```python
from build123d import *

# Parameters (mm, degrees)
F0_R     = 1.494135
F1_DEPTH = 2.54


with BuildPart() as f1:
    # F0 (on Top) → F1 (new body)
    with BuildSketch(Plane.XY):
        with BuildLine():
            Line((13.48222, 2.024483), (3.201543, 2.496718))
            Line((3.201543, 2.496718), (0.474253, 11.350792))
            ThreePointArc((0.474253, 11.350792), (0.005987, 16.463631), (-0.486017, 11.353022))
            Line((-0.486017, 11.353022), (-3.337723, 2.332209))
            Line((-3.337723, 2.332209), (-13.398782, 1.982259))
            Line((-13.398782, 1.982259), (-5.530131, -4.593079))
            Line((-5.530131, -4.593079), (-8.383425, -15.383421))
            Line((-8.383425, -15.383421), (-8.195174, -15.200495))
            Line((-8.195174, -15.200495), (0, -9.12891))
            Line((0, -9.12891), (8.333031, -15.200495))
            Line((8.333031, -15.200495), (5.491082, -4.593079))
            Line((5.491082, -4.593079), (5.580035, -4.494939))
            Line((5.580035, -4.494939), (13.48222, 2.024483))
        make_face()
        Polygon((-0.515748, -8.972427), (-7.396878, -14.017268), (-0.785596, -2.886029), (-0.214107, -8.758916), align=None, mode=Mode.SUBTRACT)
        Polygon((-12.247529, 1.427319), (-1.096065, -2.263094), (-5.187609, -4.228639), align=None, mode=Mode.SUBTRACT)
        Polygon((4.948679, -4.494939), (7.647161, -14.017268), (0, -2.683643), align=None, mode=Mode.SUBTRACT)
        Polygon((11.950911, 1.767228), (0, -1.88404), (3.035744, 1.982259), align=None, mode=Mode.SUBTRACT)
        Polygon((-2.941626, 2.241765), (-0.236567, 11.293307), (-0.65273, -1.555721), align=None, mode=Mode.SUBTRACT)
        with Locations((0, 13.88522)):
            Circle(F0_R, mode=Mode.SUBTRACT)
    extrude(amount=F1_DEPTH)


solid = f1.part
```
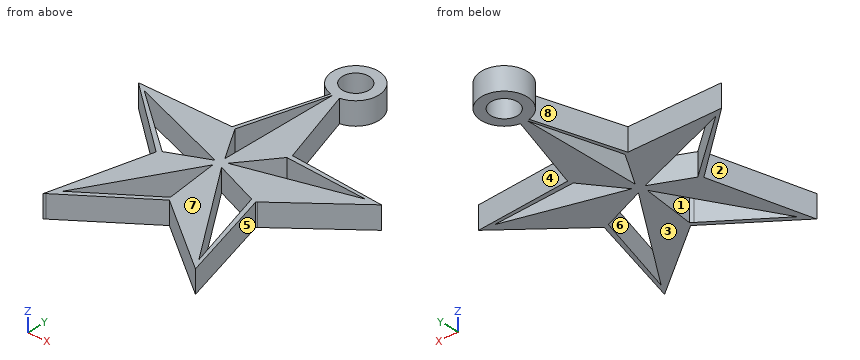
Can you work these out from the model? Positions are in its coordinate system, mm. Face numbers are marked on the shaded views. A direction names the side the tool comes from. Coordinates: 2 decimals unless noted, no trailing zeros. Loops run counter-clockwise (first coordinate to the right, second up) from the corner with the lowest first, then second, coordinate; pieces in that order, holes last. Notation, with made-up numbers: (-25.75, -34.75) -> (24.25, -34.75) arc R17 ccw to (24.25, -18.75) -> close; hole circle Ø4 at (-3.75, 56). An arc over 180 degrees is marked (long way). Answer as a JSON object with one key per item and string values.
1) Thinking about a two-plate mould opening in X: for the marked faces 6, 7 and 8, which applies, pulls with the +X half, pulls with the -X half, needs draft (parallel to the pull), parting line crosses it, or undercut?
Results:
{"face 6": "undercut", "face 7": "needs draft", "face 8": "pulls with the -X half"}
2) Imagine slicing it at C-C (z = 1.35). Count the separate pieces of the cut face and the enclosed holes in it, then the cut area to 3 significant figures.
Results:
{"separate pieces": "1", "enclosed holes": "6", "area": "181 mm^2"}
3) Imagine slicing it at D-D (x = -6.25). Please give me the cut outline in (y, z).
Results:
{"outline": "(-13.76, 0) -> (-13.18, 0) -> (-13.18, 2.54) -> (-13.76, 2.54) -> close; (-12.09, 0) -> (-7.32, 0) -> (-7.32, 2.54) -> (-12.09, 2.54) -> close; (-3.99, 0) -> (-3.38, 0) -> (-3.38, 2.54) -> (-3.99, 2.54) -> close; (-0.56, 0) -> (2.23, 0) -> (2.23, 2.54) -> (-0.56, 2.54) -> close"}
4) If I drill on line 1 (X direction, y = 14, z = 0.85); line 2 (Y direction, x = -3.75, z = 2.15); line 3 (X direction, y = -10, z = 1.65), over which ranges is the centre line in solid material (lowest first)?
Results:
{"line 1": "x = -2.58 to -1.49, 1.49 to 2.58", "line 2": "y = -11.91 to -11.34, -7.88 to -3.54, -1.38 to 2.32", "line 3": "x = -6.96 to -5.01, -1.92 to -1.18, 1.2 to 4.94, 6.51 to 6.94"}
5) For P1, Ø1.5, axis at x = 10, y = 3, coming from the +Z side; P2, Ø10, axis at x = -3, y = -4.5, coming from the -Z side; P3, Ø1, axis at y = -10.5, z = 2, coming from the -X side, each with a flat end and sliding along its axis, tell me the tip position at first contact or that it passes through.
Results:
{"P1": "passes through", "P2": "stops at z = 0", "P3": "stops at x = -7.22"}
6) Imagine slicing it at A-A (x = -10.75). Please give me the cut outline in (y, z), then the cut area to 3 significant figures.
Results:
{"outline": "(-0.23, 0) -> (0.23, 0) -> (0.23, 2.54) -> (-0.23, 2.54) -> close; (0.93, 0) -> (2.07, 0) -> (2.07, 2.54) -> (0.93, 2.54) -> close", "area": "4.07 mm^2"}
7) Imagine slicing it at B-B (y = -3.5). Please give me the cut outline in (x, z), then the cut area to 3 significant figures.
Results:
{"outline": "(-6.84, 0) -> (-6.1, 0) -> (-6.1, 2.54) -> (-6.84, 2.54) -> close; (-3.67, 0) -> (-1.15, 0) -> (-1.15, 2.54) -> (-3.67, 2.54) -> close; (-0.73, 0) -> (0.55, 0) -> (0.55, 2.54) -> (-0.73, 2.54) -> close; (2.23, 0) -> (6.79, 0) -> (6.79, 2.54) -> (2.23, 2.54) -> close", "area": "23.1 mm^2"}
8) For the marked faces 1, 2, 3, 4 and 5, which set-ups out of +Z, -Z, +X, -X, +Y, -Y let a thin tool reach every point of the face, with its end or its side?
Results:
{"face 1": "+Z, -Z", "face 2": "+Z, -Z, -X", "face 3": "-Z, +X, -X, +Y, -Y", "face 4": "+Z, -Z, +X, +Y", "face 5": "+Z, -Z, +X"}
